The model under review builds one solid part; all positions refer to its coordinate system, in mm. A direction names the side the tool comes from. Round coordinates to 2 decimals unless told otherwise and drop trailing zeros. Order: outer loops, then holes, each group sorted by start corner. A loop starts at its lowest first (then second) coordinate and runs counter-clockwise, first axis right, second up. Notation, with made-up numbers: M 67,49.5 L 116,49.5 A20 cw 116,80.5 Z; hole C 43,-27.75 d9. An arc over 180 degrees is marked long. Use a Markdown table: item, result. Add a question column.
1. To check wall thickness, follow probe 1 along Y at (x, z) = (-6.1, 0); probe 2 along Y at (x, z) = (-7, 1.25); probe 3 along Z at (x, y) = (4, 12). State the ranges of each line that lie inside material, in increasing order.
2. Consider section B-B on z = 0. State the section outline as (x, y) points, then the cut area to 3 significant figures.
3. For faces 1 (the cylindrical face through (-8.584, 9.86, -2.703)), 2 (the cylindrical face through (4.619, 15.07, 1.915)), list the 3-axis set-ups (+Z, -Z, +X, -X, +Y, -Y) from which the entire face can be reached by the end or side of a thin tool; tool diameter is ignored.
4. The part is to be moulded in two halves that separate along Y. For faces 3 (the flat face through (-4, 20, -4)), 4 (the cylindrical face through (-6.04, 3.5, 0.07)), 5 (the flat face through (0, 0, -4)), 6 (the cylindrical face through (-6.855, 14.675, -1.464)), say which applies: +Y half, -Y half, draft (parallel to the pull), parting line (faces both ways), or undercut.
5. Consider section A-A on x = 0. State the section outline as (y, z) points.
6. Consider section C-C on y = 5. State the section outline as (x, z) points.
7. Consider section D-D on y = 9.25. State the section outline as (x, z) points.
8. Insertion check: P1, Ø4, axis at x = 4, y = 12.5, coming from the +Z side; P2, Ø1.8, axis at y = 15, z = 0, coming from the +X side; P3, Ø4, axis at x = -3.5, y = 14.5, coming from the +Z side; P4, Ø9, axis at x = 0, z = 0, coming from the +Y side. Each pin has a flat end and moves straight along its axis. Give the tip position at first contact, or say it passes through.
Autodesk Inventor part; units mm, degrees
ref_plane "YZ Plane" through (0, 0, 0) normal (1, 0, 0) x (0, 1, 0)
ref_plane "XZ Plane" through (0, 0, 0) normal (0, 1, 0) x (-1, 0, 0)
ref_plane "XY Plane" through (0, 0, 0) normal (0, 0, 1) x (1, 0, 0)
sketch "Эскиз1" plane through (0, 0, 0) normal (0, 1, 0) x (-1, 0, 0)
  circle A0 centre (0, 0) radius 3.5
  circle A1 centre (0, 0) radius 9
  dimension "d0" = 7
  dimension "d1" = 18
extrude "Выдавливание1" add sketch "Эскиз1" along normal blind 20
sketch "Эскиз2" plane through (0, 20, 0) normal (0, 1, 0) x (1, 0, 0)
  circle A0 centre (0, 0) radius 5
  dimension "d4" = 10
extrude "Выдавливание2" cut sketch "Эскиз2" against normal blind 10
sketch "Эскиз3" plane through (0, 0, 0) normal (1, 0, 0) x (0, 1, 0)
  line L0 (20, -9) -> (20, 9)
  line L1 (20, 0) -> (15, 0)
  line L2 (0, 0) -> (5, 0)
  circle A0 centre (15, 0) radius 1.5
  circle A1 centre (5, 0) radius 1.5
  dimension "d7" = 5
  dimension "d8" = 5
  dimension "d9" = 3
  dimension "d10" = 3
extrude "Выдавливание3" cut sketch "Эскиз3" along normal mid plane 27.5
thread "Резьба1"
thread "Резьба2"
sketch "Эскиз4" plane through (0, 0, 0) normal (0, 0, 1) x (1, 0, 0)
  line L0 (3.5, 10) -> (3.5, 0)
  line L1 (-5, 10) -> (5, 10)
  line L2 (-3.5, 10) -> (-3.5, 0)
  line L3 (-9, 6.5) -> (-3.5, 6.5)
  line L4 (-9, 3.5) -> (-3.5, 3.5)
  line L5 (3.5, 3.5) -> (9, 3.5)
  line L6 (3.5, 6.5) -> (9, 6.5)
  line L7 (-3.5, 5) -> (3.5, 5)
  line L8 (0, 5) -> (0, 0)
properties part number "Втулка энкодер"
Answer block:
| question | item | result |
|---|---|---|
| 1 | probe 1 | 0 to 3.5, 6.5 to 13.5, 16.5 to 20 |
| 1 | probe 2 | 0 to 4.17, 5.83 to 14.17, 15.83 to 20 |
| 1 | probe 3 | -8.06 to -3, 3 to 8.06 |
| 2 | outline | M -9,0 L -3.5,0 L -3.5,3.5 L -9,3.5 Z; M -9,6.5 L -3.5,6.5 L -3.5,10 L -5,10 L -5,13.5 L -9,13.5 Z; M -9,16.5 L -5,16.5 L -5,20 L -9,20 Z; M 3.5,0 L 9,0 L 9,3.5 L 3.5,3.5 Z; M 3.5,6.5 L 9,6.5 L 9,13.5 L 5,13.5 L 5,10 L 3.5,10 Z; M 5,16.5 L 9,16.5 L 9,20 L 5,20 Z |
| 2 | area | 133 mm^2 |
| 3 | face 1 | +Y, -Y |
| 3 | face 2 | +Y |
| 4 | face 3 | +Y half |
| 4 | face 4 | undercut |
| 4 | face 5 | -Y half |
| 4 | face 6 | undercut |
| 5 | outline | M 0,-9 L 20,-9 L 20,-5 L 10,-5 L 10,-3.5 L 0,-3.5 Z; M 0,3.5 L 10,3.5 L 10,5 L 20,5 L 20,9 L 0,9 Z |
| 6 | outline | M -8.87,-1.5 A9 ccw 8.87,-1.5 L 3.16,-1.5 A3.5 cw -3.16,-1.5 Z; M -8.87,1.5 L -3.16,1.5 A3.5 cw 3.16,1.5 L 8.87,1.5 A9 ccw Z |
| 7 | outline | C 0,0 d18; hole C 0,0 d7 |
| 8 | P1 | z = 8.77 |
| 8 | P2 | through |
| 8 | P3 | z = 8.87 |
| 8 | P4 | y = 10 |
